Can you work these out from the model? Positions are in its coordinate system, mm. A direction names the side the tool comes from. Round coordinates to 2 decimals unless told otherwise and drop trailing zeros. Loops run counter-clockwise (first coordinate to the right, second up) from the corner with the lowest first, then second, coordinate; pieces in that order, holes last. Notation, with made-up numbers: (76, 23) -> (105, 23) arc R22 ccw to (105, 40) -> close; hole circle Ø8 at (9, 71). An arc over 180 degrees is marked (long way). Answer as a JSON object with one key per item and string values.
```python
from build123d import *

# Parameters (mm, degrees)
SKETCH1_W           = 75
SKETCH1_H           = 12
BOSS_EXTRUDE1_DEPTH = 10
CUT_EXTRUDE1_DEPTH  = 7
SKETCH3_R           = 10
BOSS_EXTRUDE2_DEPTH = 10
BOSS_EXTRUDE3_DEPTH = 3
FILLET1_R           = 2


with BuildPart() as part:
    # Sketch1 → Boss-Extrude1 (new body)
    with BuildSketch(Plane.XY):
        Rectangle(SKETCH1_W, SKETCH1_H)
    extrude(amount=BOSS_EXTRUDE1_DEPTH)

    # Sketch2 → Cut-Extrude1 (cut)
    with BuildSketch(Plane.XY.offset(10)):
        Polygon((0, -7.505553499), (6.5, -3.75277675), (6.5, 3.75277675), (0, 7.505553499), (-6.5, 3.75277675), (-6.5, -3.75277675), align=None)
    extrude(amount=-CUT_EXTRUDE1_DEPTH, mode=Mode.SUBTRACT)

    # Sketch3 → Boss-Extrude2 (add)
    with BuildSketch(Plane(origin=(0, 0, 0), x_dir=(-1, 0, 0), z_dir=(0, 0, -1))):
        Circle(SKETCH3_R)
        Polygon((0, -7.505553499), (6.5, -3.75277675), (6.5, 3.75277675), (0, 7.505553499), (-6.5, 3.75277675), (-6.5, -3.75277675), align=None, mode=Mode.SUBTRACT)
    extrude(amount=-BOSS_EXTRUDE2_DEPTH)

    # Sketch4 → Boss-Extrude3 (add)
    with BuildSketch(Plane(origin=(0, 0, 0), x_dir=(-1, 0, 0), z_dir=(0, 0, -1))):
        Polygon((2.607695155, 6), (0, 7.505553499), (-2.607695155, 6), align=None)
        Polygon((0, -7.505553499), (2.607695155, -6), (-2.607695155, -6), align=None)
    extrude(amount=-BOSS_EXTRUDE3_DEPTH)

    # Fillet1
    fillet1_edges = [part.edges().sort_by_distance(p)[0] for p in [
        (-37.5, 0, 10),
        (-22.75, -6, 10),
        (37.5, 0, 10),
        (-22.75, -6, 0),
        (22.75, -6, 0),
        (-22.75, 6, 0),
        (-37.5, 0, 0),
        (22.75, -6, 10),
        (22.75, 6, 0),
        (-22.75, 6, 10),
        (0, 10, 0),
        (0, -10, 0),
        (0, 10, 10),
        (37.5, 0, 0),
        (-8, 6, 5),
        (-8, -6, 5),
        (0, -10, 10),
        (8, 6, 5),
        (8, -6, 5),
        (22.75, 6, 10),
        (37.5, -6, 5),
        (-37.5, -6, 5),
        (-37.5, 6, 5),
        (37.5, 6, 5),
    ]]
    fillet(fillet1_edges, radius=FILLET1_R)


solid = part.part
```
Q1. I want a section at B-B, the plane y = -2. Write out the boundary of the cut face in (x, z).
Determined:
{"outline": "(-37.5, 2) arc R2 ccw to (-35.5, 0) -> (35.5, 0) arc R2 ccw to (37.5, 2) -> (37.5, 8) arc R2 ccw to (35.5, 10) -> (6.5, 10) -> (6.5, 3) -> (-6.5, 3) -> (-6.5, 10) -> (-35.5, 10) arc R2 ccw to (-37.5, 8) -> close"}
Q2. We'd pull the mould along Y, two halves only. Please class faces 6 (the flat face through (-8, 0, 10)), 7 (the flat face through (3.2, 5.66, 6.45)), 8 (the flat face through (-6.5, 0, 7)), 9 (the cylindrical face through (-22.04, 5.4, 0.57)): pulls with the +Y half, pulls with the -Y half, needs draft (parallel to the pull), parting line crosses it, or undercut.
Determined:
{"face 6": "needs draft", "face 7": "undercut", "face 8": "undercut", "face 9": "pulls with the +Y half"}
Q3. I want a section at A-A, the plane z = 6. Write out the boundary of the cut face in (x, y).
Determined:
{"outline": "(-37.5, -4) arc R2 ccw to (-35.5, -6) -> (-8.94, -6) arc R2 cw to (-7.45, -6.67) arc R10 ccw to (7.45, -6.67) arc R2 cw to (8.94, -6) -> (35.5, -6) arc R2 ccw to (37.5, -4) -> (37.5, 4) arc R2 ccw to (35.5, 6) -> (8.94, 6) arc R2 cw to (7.45, 6.67) arc R10 ccw to (-7.45, 6.67) arc R2 cw to (-8.94, 6) -> (-35.5, 6) arc R2 ccw to (-37.5, 4) -> close; hole (-6.5, -3.75) -> (0, -7.51) -> (6.5, -3.75) -> (6.5, 3.75) -> (0, 7.51) -> (-6.5, 3.75) -> close"}
Q4. If I drill on L1, parallel to X at y = 3, z = 4.75; L2, parallel to Z at x = 34, y = 4.25; L3, parallel to Y at x = 18, z = 2.25, over which ranges is the centre line in solid material (lowest first)? Write a range as [from, to].
Determined:
{"L1": "[-37.5, -6.5], [6.5, 37.5]", "L2": "[0.02, 9.98]", "L3": "[-6, 6]"}
Q5. I want a section at C-C, the plane x = 18.5. Write out the boundary of the cut face in (y, z).
Determined:
{"outline": "(-6, 2) arc R2 ccw to (-4, 0) -> (4, 0) arc R2 ccw to (6, 2) -> (6, 8) arc R2 ccw to (4, 10) -> (-4, 10) arc R2 ccw to (-6, 8) -> close"}
Q6. I'm going to push flat-ended pins straight in: pin 1 (1 mm diameter, centred on y = 5, z = 6.5, fed in from -X); pin 2 (3 mm diameter, centred on x = 19, z = 5.5, fed in from -Y); pin 3 (1 mm diameter, centred on x = 0, y = -6.5, fed in from +Z). Where does each tip first touch, or does it pass through?
Determined:
{"pin 1": "x = -37.44", "pin 2": "y = -6", "pin 3": "z = 3"}
Q7. On a 3-axis mill with a long thin cutter (end or side, diameter ignored), from which of +Z, -Z, +X, -X, +Y, -Y can I reach the whole of each face in a straight line? I mean faces 1 (the flat face through (6.5, 0, 7)), 2 (the flat face through (22, -6, 5)), 3 (the cylindrical face through (-22.04, -5.4, 0.57)), 4 (the cylindrical face through (22.41, -5.43, 9.4)), 5 (the cylindrical face through (-22.04, 5.43, 9.4)). Say none if no direction works.
Determined:
{"face 1": "+Z", "face 2": "+Z, -Z, +X, -Y", "face 3": "-Z, -X, -Y", "face 4": "+Z, +X, -Y", "face 5": "+Z, -X, +Y"}
